Verification items for the finished model (mm, model axes). Give positions to 0.01 mm unless a question says otherwise; leave off trailing zeros. Loops run counter-clockwise (first coordinate to the right, second up) from the corner with the lowest first, then second, coordinate; pieces in that order, holes last. Notation, with made-up numbers: M 57.25,28.25 L 107.25,28.25 A8 cw 107.25,35.25 Z; hole C 57,-21 d9. An arc over 180 degrees is marked long. Use CSV: the item, a comma, the result in double quotes.
from build123d import *

# Parameters (mm, degrees)
SKETCH_1_W          = 80
SKETCH_1_H          = 61
EXTRUDE_1_DEPTH     = 1.5
SKETCH_5_W          = 80
SKETCH_5_H          = 61
SKETCH_5_W_2        = 76
SKETCH_5_H_2        = 57
EXTRUDE_3_DEPTH     = 35
CUT_EXTRUDE_2_DEPTH = 108.01985797


with BuildPart() as part:
    # 草图1 → 凸台-拉伸1 (new body)
    with BuildSketch(Plane(origin=(0, 0, 0), x_dir=(1, 0, 0), z_dir=(0, 1, 0))):
        with Locations((40, 30.5)):
            Rectangle(SKETCH_1_W, SKETCH_1_H)
    extrude(amount=EXTRUDE_1_DEPTH)

    # 草图5 → 凸台-拉伸3 (add)
    with BuildSketch(Plane(origin=(0, 1.5, 0), x_dir=(1, 0, 0), z_dir=(0, 1, 0))):
        with Locations((40, 30.5)):
            Rectangle(SKETCH_5_W, SKETCH_5_H)
        with Locations((40, 30.5)):
            Rectangle(SKETCH_5_W_2, SKETCH_5_H_2, mode=Mode.SUBTRACT)
    extrude(amount=EXTRUDE_3_DEPTH)

    # 草图6 → 切除-拉伸2 (cut, through all)
    with BuildSketch(Plane.XY):
        Polygon((1, 36.5), (80, 36.5), (80, 1), align=None)
    extrude(amount=-CUT_EXTRUDE_2_DEPTH, mode=Mode.SUBTRACT)


solid = part.part
(1) Section check A-A on y = 8. Record the cut outline in (x, z), plus the area to 3 significant figures.
Calculated:
outline,"M 0,-61 L 64.42,-61 L 64.42,-59 L 2,-59 L 2,-2 L 64.42,-2 L 64.42,0 L 0,0 Z"
area,"372 mm²"
(2) Section check C-C on x = 39.5. Record the cut outline in (y, z), plus the area to 3 significant figures.
Calculated:
outline,"M 0,-61 L 19.2,-61 L 19.2,-59 L 1.5,-59 L 1.5,-2 L 19.2,-2 L 19.2,0 L 0,0 Z"
area,"162 mm²"
(3) Section check B-B on z = -41.5. Record the cut outline in (x, y), plus the area to 3 significant figures.
Calculated:
outline,"M 0,0 L 80,0 L 80,1 L 78,1.9 L 78,1.5 L 2,1.5 L 2,36.05 L 1,36.5 L 0,36.5 Z"
area,"190 mm²"
(4) Depth check by flat-ended pin: pin 1 Ø8 at (x, z) = (19.5, -45.5) entering from +Y. Enter the tip coordinate at first touch or a pass-through.
Calculated:
pin 1,"stops at y = 1.5"
(5) Mould release check, pull along X, two halves, no side actions. Record for faces 1 (the flat face through (78.721, 1.575, -30.358)), 2 (the flat face through (0, 18, -30)), 3 (the flat face through (31, 14, 0)), 4 (the flat face through (39, 1.5, -31)): released by +X, released by -X, zero draft, split by the parting line, or undercut.
Calculated:
face 1,"released by +X"
face 2,"released by -X"
face 3,"zero draft"
face 4,"undercut"
(6) Scan lines: L1, parallel to Z at x = 9, y = 25; L2, parallel to Y at x = 6, z = -49.5; L3, parallel to X at y = 8, z = -22. Record each from-to range of solid material in increasing order. Write a range as from..to.
Calculated:
L1,"z = -61..-59, -2..0"
L2,"y = 0..1.5"
L3,"x = 0..2"
